Autodesk Inventor part; units mm, degrees
ref_plane "YZ Plane" through (0, 0, 0) normal (1, 0, 0) x (0, 1, 0)
ref_plane "XZ Plane" through (0, 0, 0) normal (0, 1, 0) x (-1, 0, 0)
ref_plane "XY Plane" through (0, 0, 0) normal (0, 0, 1) x (1, 0, 0)
sketch "草图2" plane through (0, 0, 0) normal (0, 0, 1) x (1, 0, 0)
  line L0 (-0.6667, -13.4014) -> (-4.2667, -13.4014)
  line L1 (-0.6667, -9.4014) -> (-0.6667, -13.4014)
  arc A0 (0.6667, -9.4014) -> (-0.6667, -9.4014) centre (0, 0) ccw
  arc A1 (7.2634, -7.604) -> (-7.2634, -7.604) centre (0, 0.8667) ccw
  line L2 (0, -19.4467) -> (0, 17.2703)
  line L3 (0.6667, -13.4014) -> (4.2667, -13.4014)
  line L4 (0.6667, -9.4014) -> (0.6667, -13.4014)
  arc A2 (-4.2667, -13.4014) -> (-7.2634, -7.604) centre (-12.9205, -14.2014) ccw
  arc A3 (7.2634, -7.604) -> (4.2667, -13.4014) centre (12.9205, -14.2014) ccw
  dimension "d15" = 0.8667
  dimension "d28" = 18.85
  dimension "d32" = 2.6
  dimension "d34" = 4
  dimension "d35" = 1.3333
  dimension "d48" = 3.6
  dimension "d49" = 0.8
extrude "拉伸1" add sketch "草图2" against normal blind 1.1
sketch "草图3" plane through (0, 0, 0) normal (0, 0, 1) x (1, 0, 0)
  circle A0 centre (-2.5667, -11.4014) radius 1
  line L0 (-0.6667, -13.4014) -> (-4.2667, -13.4014)
  line L1 (0.6667, -13.4014) -> (0.6667, -9.4014)
  line L2 (4.2667, -13.4014) -> (0.6667, -13.4014)
  line L3 (0, -14.2014) -> (0, -8.6014)
  circle A1 centre (2.5667, -11.4014) radius 1
  dimension "d36" = 2
  dimension "d37" = 2
  dimension "d47" = 5.1333
extrude "拉伸2" cut sketch "草图3" against normal through all
equation "\"d15\" = 0.333333 * b"
equation "\"d28\" = g1"
equation "\"d32\" = b"
equation "\"d34\" = ParA"
equation "\"d35\" = 0.333333 * ParA"
equation "\"d48\" = 1.8 * Diam5"
equation "\"d49\" = 0.2 * ParA"
equation "\"d16\" = tt"
equation "\"d36\" = Diam5"
equation "\"d37\" = 0.5 * ParA"
equation "\"d47\" = 0.333333 * ParA + 1.9 * Diam5"
equation "\"g1\" = 18.85"
equation "\"ParA\" = 4"
equation "\"tt\" = 1.1"
equation "\"Diam5\" = 2"
equation "\"TEMPLATE\" = 1.2345"
properties part number "ANSI B 27.7M - 3AMI-20" material "钢，软"
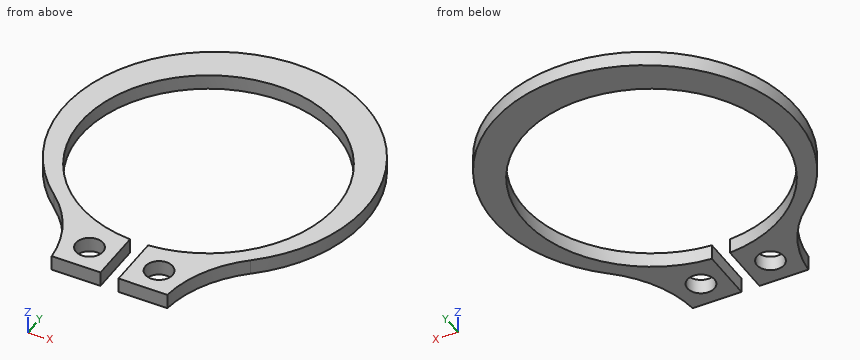
Geometry: final body of the model. Coordinates: model frame, mm. Round coordinates to 2 decimals unless told otherwise and drop trailing zeros. Loops run counter-clockwise (first coordinate to the right, second up) from the corner with the lowest first, then second, coordinate; pieces in that order, holes last. Notation, with made-up numbers: M 47.25,52.5 L 51.25,52.5 A29 cw 51.25,87.5 Z; hole C 52.5,-27 d1. An arc over 180 degrees is marked long. Put each result on its own line as item: value. Start each with the question number.
(1) Section query A-A (y = 8). Return loops of the section in (x, z), then the cut area to 3 significant figures.
(2) Section query D-D (x = -2.75). Return loops of the section in (y, z), then the cut area to 3 significant figures.
(3) Material intervals for line 1 along Y through (x, z) = (-2, -0.95); line 2 along Y through (x, z) = (-3.25, -0.65); line 3 along X through (y, z) = (-11.5, -0.9), sorted ascending. Write a range as [from, to].
(4) Section query C-C (x = -8.5). Return loops of the section in (y, z), then the cut area to 3 significant figures.
(5) Section query B-B (z = -0.55). Return loops of the section in (x, y) (3 decimals), then the cut area to 3 significant figures.
(6) Contact query for a flat-ended pin moving along its axis: pin 1 Ø1.6 at (x, y) = (2.57, -11.4) entering from -Z. Output: stop coordinate, or through.
Findings below:
1. outline: M -8.58,-1.1 L -4.98,-1.1 L -4.98,0 L -8.58,0 Z; M 4.98,-1.1 L 8.58,-1.1 L 8.58,0 L 4.98,0 Z
1. area: 7.91 mm2
2. outline: M -13.4,-1.1 L -12.38,-1.1 L -12.38,0 L -13.4,0 Z; M -10.42,-1.1 L -9.01,-1.1 L -9.01,0 L -10.42,0 Z; M 9.01,-1.1 L 11.68,-1.1 L 11.68,0 L 9.01,0 Z
2. area: 5.60 mm2
3. line 1: y = [-13.4, -12.23], [-10.58, -9.21], [9.21, 11.84]
3. line 2: y = [-13.4, -12.13], [-10.67, -8.85], [8.85, 11.54]
3. line 3: x = [-4.66, -3.56], [-1.57, -0.67], [0.67, 1.57], [3.56, 4.66]
4. outline: M -6.36,-1.1 L -4.07,-1.1 L -4.07,0 L -6.36,0 Z; M 4.07,-1.1 L 8.1,-1.1 L 8.1,0 L 4.07,0 Z
4. area: 6.95 mm2
5. outline: M -7.263,-7.604 A8.691 cw -4.267,-13.401 L -0.667,-13.401 L -0.667,-9.401 A9.425 cw long 0.667,-9.401 L 0.667,-13.401 L 4.267,-13.401 A8.691 cw 7.263,-7.604 A11.158 ccw long Z; hole C -2.567,-11.401 d2; hole C 2.567,-11.401 d2
5. area: 135 mm2
6. pin 1: passes through
